Design review of the part built by this model. Coordinates are the model's own, in mm. Face numbers are marked on the shaded views. A direction names the side the tool comes from. Give positions to 0.01 mm unless a question says otherwise; leave off trailing zeros. Order: outer loops, then holes, each group sorted by start corner. A loop starts at its lowest first (then second) coordinate and runs counter-clockwise, first axis right, second up. Notation, with made-up numbers: (-36, -30.5) -> (6, -30.5) arc R22 ccw to (6, -4.5) -> close; hole circle Ø4 at (22.5, -2). An arc over 180 degrees is marked (long way). One line per item, written item: value. Start each with the question number.
1) For pin 1 (3 mm diameter, centred on x = 11, y = 25.5, fed in from +Z); pin 2 (4 mm diameter, centred on y = 35.59, z = 19.42, fed in from -X); pin 3 (7.5 mm diameter, centred on y = 30.5, z = 10.5, fed in from +X); pin 4 (4 mm diameter, centred on x = 16, z = 21, fed in from +Y), all flat-tipped, find the tip position at first contact; note any pin that passes through.
2) Consider section C-C (y = 19.5). State the section outline as (x, z) points, plus the area to 4 significant figures.
3) Consider section A-A (y = -16.5). State the section outline as (x, z) points.
4) Tool access review of the marked faces 1, 2 and 3: name each direction out of +Z, -Z, +X, -X, +Y, -Y from which nothing blocks a thin tool from reaching the whole face with its end or side.
5) Consider section D-D (x = 16). State the section outline as (y, z) points.
6) Consider section B-B (z = 16). State the section outline as (x, y) points, plus the area to 3 significant figures.
7) The part is to be moulded in two halves that separate along X. For the marked faces 4, 5 and 6, say which applies: released by +X, released by -X, zero draft, split by the parting line, or undercut.
8) Wall thickness on line 1 along X through (y, z) = (-16.5, 22.25); line 2 along Y through (x, z) = (7.5, 18.5); line 3 along Y through (x, z) = (7.5, 18.75): over which ranges is each line inside the solid? List them lowest first. Write a range as from..to.
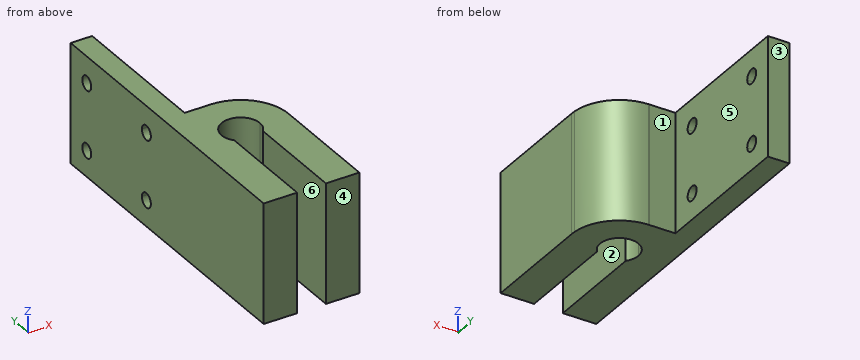
from build123d import *

# Parameters (mm, degrees)
F1_DEPTH      = 25
F3_DEPTH      = 25
F3_DEPTH_BACK = 25


with BuildPart() as f1:
    # F0 (on Top) → F1 (new body)
    with BuildSketch(Plane.XY):
        with BuildLine():
            Line((3.69989, 0), (3.69989, -23.748155))
            Line((3.69989, -23.748155), (10.309355, -23.748155))
            Line((10.309355, -23.748155), (10.69989, -23.748155))
            Line((10.69989, -23.748155), (10.69989, -2.645751))
            ThreePointArc((10.69989, -2.645751), (9.958232, -1.414214), (9.69989, 0))
            Line((9.69989, 0), (3.69989, 0))
        make_face()
        with BuildLine():
            ThreePointArc((3.74811, 0.980861), (3.711952, 0.491023), (3.69989, 0))
            Line((3.69989, 0), (9.69989, 0))
            ThreePointArc((9.69989, 0), (13.69989, 4), (17.69989, 0))
            Line((17.69989, 0), (23.69989, 0))
            ThreePointArc((23.69989, 0), (23.687827, 0.491023), (23.651669, 0.980861))
            ThreePointArc((23.651669, 0.980861), (20.450878, 7.377273), (13.796338, 9.999535))
            Line((13.796338, 9.999535), (13.603441, 9.999535))
            Line((13.603441, 9.999535), (8.19989, 9.999535))
            Line((8.19989, 9.999535), (8.19989, 40.999535))
            Line((8.19989, 40.999535), (3.69989, 40.999535))
            Line((3.69989, 40.999535), (3.69989, 23.748155))
            Line((3.69989, 23.748155), (3.69989, 9.999535))
            Line((3.69989, 9.999535), (3.69989, 0.980861))
            Line((3.69989, 0.980861), (3.74811, 0.980861))
        make_face()
        with BuildLine():
            Line((3.69989, 0.980861), (3.69989, 0))
            ThreePointArc((3.69989, 0), (3.711952, 0.491023), (3.74811, 0.980861))
            Line((3.74811, 0.980861), (3.69989, 0.980861))
        make_face()
        with BuildLine():
            Line((23.69989, 0), (17.69989, 0))
            ThreePointArc((17.69989, 0), (17.441547, -1.414214), (16.69989, -2.645751))
            Line((16.69989, -2.645751), (16.69989, -23.748155))
            Line((16.69989, -23.748155), (23.69989, -23.748155))
            Line((23.69989, -23.748155), (23.69989, 0))
        make_face()
        with BuildLine():
            Line((13.603441, 9.999535), (13.796338, 9.999535))
            ThreePointArc((13.796338, 9.999535), (13.69989, 10), (13.603441, 9.999535))
        make_face()
    extrude(amount=F1_DEPTH)

    # F2 (on face) → F3 (cut, two sides)
    with BuildSketch(Plane(origin=(3.69989, 0, 0), x_dir=(0, -1, 0), z_dir=(-1, 0, 0))) as f3_sk:
        with BuildLine():
            Line((-15.599724, 5.426402), (-17.099724, 5.426402))
            ThreePointArc((-17.099724, 5.426402), (-15.599724, 3.926402), (-14.099724, 5.426402))
            ThreePointArc((-14.099724, 5.426402), (-14.539063, 6.487062), (-15.599724, 6.926402))
            Line((-15.599724, 6.926402), (-15.599724, 5.426402))
        make_face()
        with BuildLine():
            Line((-34.08602, 5.426402), (-35.58602, 5.426402))
            Line((-35.58602, 5.426402), (-35.58602, 6.926402))
            ThreePointArc((-35.58602, 6.926402), (-36.64668, 4.365742), (-34.08602, 5.426402))
        make_face()
        with BuildLine():
            Line((-15.599724, 19.423114), (-15.599724, 17.923114))
            ThreePointArc((-15.599724, 17.923114), (-14.539063, 18.362454), (-14.099724, 19.423114))
            ThreePointArc((-14.099724, 19.423114), (-15.599724, 20.923114), (-17.099724, 19.423114))
            Line((-17.099724, 19.423114), (-15.599724, 19.423114))
        make_face()
        with BuildLine():
            ThreePointArc((-17.099724, 19.423114), (-16.660384, 18.362454), (-15.599724, 17.923114))
            Line((-15.599724, 17.923114), (-15.599724, 19.423114))
            Line((-15.599724, 19.423114), (-17.099724, 19.423114))
        make_face()
        with BuildLine():
            Line((-35.58602, 19.423114), (-35.58602, 17.923114))
            ThreePointArc((-35.58602, 17.923114), (-34.52536, 18.362454), (-34.08602, 19.423114))
            Line((-34.08602, 19.423114), (-35.58602, 19.423114))
        make_face()
        with BuildLine():
            ThreePointArc((-34.08602, 19.423114), (-36.64668, 20.483774), (-35.58602, 17.923114))
            Line((-35.58602, 17.923114), (-35.58602, 19.423114))
            Line((-35.58602, 19.423114), (-34.08602, 19.423114))
        make_face()
        with BuildLine():
            Line((-35.58602, 6.926402), (-35.58602, 5.426402))
            Line((-35.58602, 5.426402), (-34.08602, 5.426402))
            ThreePointArc((-34.08602, 5.426402), (-34.52536, 6.487062), (-35.58602, 6.926402))
        make_face()
        with BuildLine():
            ThreePointArc((-15.599724, 6.926402), (-16.660384, 6.487062), (-17.099724, 5.426402))
            Line((-17.099724, 5.426402), (-15.599724, 5.426402))
            Line((-15.599724, 5.426402), (-15.599724, 6.926402))
        make_face()
    extrude(amount=F3_DEPTH, mode=Mode.SUBTRACT)
    extrude(f3_sk.sketch, amount=-F3_DEPTH_BACK, mode=Mode.SUBTRACT)


solid = f1.part
Checked values:
1. pin 1: passes through
1. pin 2: stops at x = 3.7
1. pin 3: stops at x = 8.2
1. pin 4: stops at y = 10
2. outline: (3.7, 0) -> (8.2, 0) -> (8.2, 25) -> (3.7, 25) -> close
2. area: 112.5 mm^2
3. outline: (3.7, 0) -> (10.7, 0) -> (10.7, 25) -> (3.7, 25) -> close; (16.7, 0) -> (23.7, 0) -> (23.7, 25) -> (16.7, 25) -> close
4. face 1: +Z, -Z, +X, +Y
4. face 2: +Z, -Z, -Y
4. face 3: +Z, -Z, +X, -X, +Y
5. outline: (3.27, 0) -> (9.73, 0) -> (9.73, 25) -> (3.27, 25) -> close
6. outline: (3.7, -23.75) -> (10.7, -23.75) -> (10.7, -2.65) arc R4 cw to (9.7, 0) arc R4 cw to (17.7, 0) arc R4 cw to (16.7, -2.65) -> (16.7, -23.75) -> (23.7, -23.75) -> (23.7, 0) arc R10 ccw to (23.65, 0.98) arc R10 ccw to (13.8, 10) arc R10 ccw to (13.6, 10) -> (8.2, 10) -> (8.2, 41) -> (3.7, 41) -> close
6. area: 622 mm^2
7. face 4: zero draft
7. face 5: released by +X
7. face 6: undercut
8. line 1: x = 3.7..10.7, 16.7..23.7
8. line 2: y = -23.75..14.42, 16.78..34.4, 36.77..41
8. line 3: y = -23.75..14.26, 16.94..34.25, 36.93..41
